The listing builds one solid part. Answer for the finished solid, in the listing's coordinates (mm). A direction names the side the tool comes from. Coordinates: 2 decimals unless noted, no trailing zeros. Loops run counter-clockwise (first coordinate to the right, second up) from the corner with the lowest first, then second, coordinate; pieces in that order, holes last. Notation, with made-up numbers: M 3.5,-28 L 50.5,-28 A18 ccw 50.5,-22 Z; hole C 56,78.25 d7. An arc over 180 degrees is marked long. Answer as CSV lines item,"result". Start each with the question number.
```python
from build123d import *

# Parameters (mm, degrees)
F0_W     = 20
F0_H     = 20
F1_DEPTH = 60
F2_W     = 16
F2_H     = 16
F3_DEPTH = 25
F4_R     = 5
F5_DEPTH = 25
F6_W     = 16
F6_H     = 16
F7_DEPTH = 35


with BuildPart() as f1:
    # F0 (on Front) → F1 (new body)
    with BuildSketch(Plane.XZ):
        with Locations((-5.841036, 5.892225)):
            Rectangle(F0_W, F0_H)
    extrude(amount=F1_DEPTH)

    # F2 (on face) → F3 (cut)
    with BuildSketch(Plane(origin=(0, 0, 0), x_dir=(-1, 0, 0), z_dir=(0, 1, 0))):
        with Locations((5.841036, 5.892225)):
            Rectangle(F2_W, F2_H)
    extrude(amount=-F3_DEPTH, mode=Mode.SUBTRACT)

    # F4 (on face) → F5 (cut)
    with BuildSketch(Plane(origin=(0, 0, 13.892225), x_dir=(1, 0, 0), z_dir=(0, 0, -1))):
        with Locations((-5.841036, 12.5)):
            Circle(F4_R)
    extrude(amount=F5_DEPTH, mode=Mode.SUBTRACT)

    # F6 (on face) → F7 (cut, through all)
    with BuildSketch(Plane(origin=(0, -25, 0), x_dir=(-1, 0, 0), z_dir=(0, 1, 0))):
        with Locations((5.841036, 5.892225)):
            Rectangle(F6_W, F6_H)
    extrude(amount=-F7_DEPTH, mode=Mode.SUBTRACT)


solid = f1.part
```
Item 1: For a pull along Z with two mould halves and no side action, classify faces 1 (the face through (-6, -30, -4.108)), 2 (the face through (3, 0, 6)), 3 (the face through (-6, -30, -2.108)) as pulls with the +Z half, pulls with the -Z half, needs draft (parallel to the pull), parting line crosses it, or undercut.
Item 2: For faces 4 (the face through (-6.492, -17.457, -3.094)), 5 (the face through (-13.841, -30, 6)), 6 (the face through (3, -60, 6)), determine the directions among +Z, -Z, +X, -X, +Y, -Y from which every point of the face is accessible in a straight line to the end or side of a thin tool.
Item 3: Section D-D on y = -12.5 is taken. Determine the outline of the cut face in (x, z), then the cut area to 3 significant figures.
Item 4: Section A-A on z = -1.5 is taken. Determine the outline of the cut face in (x, y), then the cut area to 3 significant figures.
Item 5: Section C-C on x = -7.5 is taken. Determine the outline of the cut face in (y, z).
Item 6: Consider line 1 (Z direction, x = -9.5, y = -53); line 2 (X direction, y = -11.5, z = 4.25); line 3 (Z direction, x = -8.5, y = -11.5). Determine where each line is inside the solid, lowest interval first.
Item 7: Section B-B on y = -28.5 is taken. Determine the outline of the cut face in (x, z).
Results are:
1,face 1,"pulls with the -Z half"
1,face 2,"needs draft"
1,face 3,"undercut"
2,face 4,"-Z"
2,face 5,"+Y, -Y"
2,face 6,"+Z, -Z, +X, -X, -Y"
3,outline,"M -15.84,-4.11 L -10.84,-4.11 L -10.84,-2.11 L -13.84,-2.11 L -13.84,13.89 L 2.16,13.89 L 2.16,-2.11 L -0.84,-2.11 L -0.84,-4.11 L 4.16,-4.11 L 4.16,15.89 L -15.84,15.89 Z"
3,area,"124 mm²"
4,outline,"M -15.84,-60 L -13.84,-60 L -13.84,0 L -15.84,0 Z; M 2.16,-60 L 4.16,-60 L 4.16,0 L 2.16,0 Z"
4,area,"240 mm²"
5,outline,"M -60,-4.11 L -17.22,-4.11 L -17.22,-2.11 L -60,-2.11 Z; M -60,13.89 L 0,13.89 L 0,15.89 L -60,15.89 Z; M -7.78,-4.11 L 0,-4.11 L 0,-2.11 L -7.78,-2.11 Z"
6,line 1,"-4.11 to -2.11, 13.89 to 15.89"
6,line 2,"-15.84 to -13.84, 2.16 to 4.16"
6,line 3,"13.89 to 15.89"
7,outline,"M -15.84,-4.11 L 4.16,-4.11 L 4.16,15.89 L -15.84,15.89 Z; hole M -13.84,-2.11 L 2.16,-2.11 L 2.16,13.89 L -13.84,13.89 Z"
